from build123d import *

# Parameters (mm, degrees)
SKETCH1_W               = 8
SKETCH1_H               = 8
BOSS_EXTRUDE1_DEPTH     = 3
CUT_EXTRUDE1_DEPTH      = 12.704699911
CUT_EXTRUDE1_DEPTH_BACK = 12.704699911
CUT_EXTRUDE2_DEPTH      = 11
SKETCH4_R               = 1.8
CUT_EXTRUDE3_DEPTH      = 0.8
SKETCH5_W               = 8
SKETCH5_H               = 1
BOSS_EXTRUDE2_DEPTH     = 2
FILLET1_R               = 4
CUT_EXTRUDE4_DEPTH      = 0.4
CUT_EXTRUDE5_DEPTH      = 0.4


with BuildPart() as part:
    # Sketch1 → Boss-Extrude1 (new body)
    with BuildSketch(Plane(origin=(0, 0, 0), x_dir=(1, 0, 0), z_dir=(0, 1, 0))):
        with Locations((4, 4)):
            Rectangle(SKETCH1_W, SKETCH1_H)
    extrude(amount=BOSS_EXTRUDE1_DEPTH)

    # Sketch2 → Cut-Extrude1 (cut, two sides: drawn at the far end of the back side and taken through both)
    with BuildSketch(Plane.XY.offset(-CUT_EXTRUDE1_DEPTH_BACK)):
        Polygon((0, 0), (0.6, 3), (0, 3), align=None)
        Polygon((8, 0), (7.4, 3), (8, 3), align=None)
    extrude(amount=CUT_EXTRUDE1_DEPTH + CUT_EXTRUDE1_DEPTH_BACK, mode=Mode.SUBTRACT)

    # Sketch3 → Cut-Extrude2 (cut)
    with BuildSketch(Plane(origin=(0, 0, 0), x_dir=(0, 0, -1), z_dir=(1, 0, 0))):
        Polygon((0, 0), (0.6, 3), (0, 3), align=None)
        Polygon((8, 3), (7.4, 3), (8, 0), align=None)
    extrude(amount=CUT_EXTRUDE2_DEPTH, mode=Mode.SUBTRACT)

    # Sketch4 → Cut-Extrude3 (cut)
    with BuildSketch(Plane.XZ):
        with Locations(Location((4, -3.75, 0), (0, 0, 270))):
            Circle(SKETCH4_R)
    extrude(amount=-CUT_EXTRUDE3_DEPTH, mode=Mode.SUBTRACT)

    # Sketch5 → Boss-Extrude2 (add)
    with BuildSketch(Plane.XZ):
        with Locations((4, -7.5)):
            Rectangle(SKETCH5_W, SKETCH5_H)
    extrude(amount=BOSS_EXTRUDE2_DEPTH)

    # Fillet1
    # the kernel refuses this fillet: 4 mm, written as the material it takes off along each edge
    with BuildSketch(Plane(origin=(8, -2, -16.660254038), x_dir=(0, 1, 0), z_dir=(0, 0, 1)), Plane(origin=(0, -2, 1.660254038), x_dir=(0, 1, 0), z_dir=(0, 0, -1))) as fillet1_piece_1:
        with BuildLine():
            CenterArc((4, 3.464101615), FILLET1_R, 180, 60)
            Line((0, 3.464101615), (-0.08, 3.464101615))
            Line((-0.08, 3.464101615), (-0.08, 0))
            Line((-0.08, 0), (0, -0.08))
            ThreePointArc((0, -0.08), (1, -0.08), (1.96, -0.069282032))
            Line((1.96, -0.069282032), (2, 0))
        make_face()
    extrude(amount=18.320508076, mode=Mode.SUBTRACT)

    # Sketch6 → Cut-Extrude4 (cut)
    with BuildSketch(Plane(origin=(0, 3, 0), x_dir=(1, 0, 0), z_dir=(0, 1, 0))):
        with BuildLine():
            add(Edge.make_bspline(
                [(5.284087955, 2.773445367), (5.333545491, 2.739545524), (5.432652736, 2.671614118), (5.590291823, 2.583736248), (5.752942084, 2.503846486), (5.865979951, 2.460876102), (5.92270975, 2.439310751)],
                knots=[0, 0, 0, 0, 0.994855506, 1.99357661, 2.993045438, 4, 4, 4, 4], degree=3))
            Line((5.92270975, 2.439310751), (5.628639237, 1.875208187))
            add(Edge.make_bspline(
                [(5.628639237, 1.875208187), (5.568520037, 1.893818156), (5.447325875, 1.93133395), (5.332925255, 1.986187111), (5.275273852, 2.013829982)],
                knots=[0, 0, 0, 0, 0.992113803, 2, 2, 2, 2], degree=3))
            add(Edge.make_bspline(
                [(5.275273852, 2.013829982), (5.26961656, 2.016684314), (5.253233801, 2.024950075), (5.223476786, 2.045298413), (5.178074812, 2.072724498), (5.118973761, 2.11071311), (5.045578888, 2.157800121), (4.95765273, 2.213934729), (4.856407872, 2.280704114), (4.783596416, 2.327731001), (4.744825134, 2.35277229)],
                knots=[0, 0, 0, 0, 0.241377655, 0.698997227, 1.371388316, 2.263975901, 3.376788369, 4.695767198, 6.240533187, 8, 8, 8, 8], degree=3))
            add(Edge.make_bspline(
                [(4.744825134, 2.35277229), (4.712670389, 2.339001865), (4.648050063, 2.311327899), (4.547788838, 2.27725121), (4.444978029, 2.248544986), (4.339982896, 2.224200245), (4.232359046, 2.206111381), (4.122258624, 2.192239309), (4.00937299, 2.18410397), (3.933139287, 2.183304154), (3.894664878, 2.182900495)],
                knots=[0, 0, 0, 0, 0.961025642, 1.931341354, 2.907359807, 3.893838693, 4.891829695, 5.905170566, 6.942759923, 8, 8, 8, 8], degree=3))
            add(Edge.make_bspline(
                [(3.894664878, 2.182900495), (3.821683976, 2.184676763), (3.679027131, 2.188148859), (3.471015208, 2.212756542), (3.275562804, 2.255408477), (3.091812023, 2.313667662), (2.920867424, 2.390147666), (2.761229426, 2.482594503), (2.615108223, 2.593406711), (2.480490537, 2.71918809), (2.361392609, 2.861354588), (2.257130725, 3.017424584), (2.168806746, 3.186880722), (2.097587685, 3.370615377), (2.041301668, 3.567142879), (2.002926315, 3.777850586), (1.978227581, 4.001488849), (1.975427333, 4.155321196), (1.973991801, 4.234182546)],
                knots=[0, 0, 0, 0, 1.098101164, 2.146474535, 3.146072545, 4.104420533, 5.041773038, 5.958565538, 6.874115049, 7.795336865, 8.725215067, 9.658214839, 10.614563411, 11.594512188, 12.618591104, 13.685899083, 14.813688224, 16, 16, 16, 16], degree=3))
            add(Edge.make_bspline(
                [(1.973991801, 4.234182546), (1.97543059, 4.313040679), (1.978227497, 4.466335509), (2.002757559, 4.689542909), (2.042412611, 4.899497801), (2.098124704, 5.096337583), (2.170410456, 5.279545107), (2.259079723, 5.449017762), (2.363505524, 5.605417057), (2.484015277, 5.747270094), (2.617919267, 5.874338646), (2.764464989, 5.984327234), (2.9219486, 6.078236158), (3.090996271, 6.154643933), (3.272074664, 6.212871015), (3.463805003, 6.255387163), (3.667248709, 6.280295733), (3.806454886, 6.283712517), (3.877837955, 6.285464598)],
                knots=[0, 0, 0, 0, 1.193283781, 2.319662245, 3.393996131, 4.424093603, 5.411284417, 6.369670503, 7.313761776, 8.251713527, 9.181123148, 10.102053383, 11.01932051, 11.951118596, 12.903560284, 13.893239571, 14.919681386, 16, 16, 16, 16], degree=3))
            add(Edge.make_bspline(
                [(3.877837955, 6.285464598), (3.948708316, 6.284176334), (4.086935049, 6.281663683), (4.288489067, 6.254790298), (4.478939684, 6.214016744), (4.658513444, 6.155241629), (4.826290277, 6.078911265), (4.983143341, 5.98623667), (5.128157857, 5.876434989), (5.26137487, 5.750578969), (5.380523981, 5.609215368), (5.486073462, 5.454669187), (5.572731816, 5.285035211), (5.645736122, 5.103191508), (5.700157026, 4.90736457), (5.740330715, 4.69867705), (5.764520815, 4.476471411), (5.76739165, 4.323719862), (5.768863596, 4.245400495)],
                knots=[0, 0, 0, 0, 1.078752742, 2.104017338, 3.091035458, 4.041673215, 4.975566109, 5.892967701, 6.810684895, 7.740128604, 8.678185021, 9.621404646, 10.583875016, 11.573429805, 12.6009998, 13.674031063, 14.80742018, 16, 16, 16, 16], degree=3))
            add(Edge.make_bspline(
                [(5.768863596, 4.245400495), (5.767275795, 4.16278925), (5.764189157, 4.002195454), (5.737326284, 3.768977018), (5.693780668, 3.550562854), (5.648918616, 3.41330904), (5.627036673, 3.346362034)],
                knots=[0, 0, 0, 0, 1.083667057, 2.106616435, 3.076482036, 4, 4, 4, 4], degree=3))
            add(Edge.make_bspline(
                [(5.627036673, 3.346362034), (5.607421404, 3.297050064), (5.567517691, 3.196733787), (5.488642668, 3.051933408), (5.394797316, 2.909076479), (5.321514211, 2.819296637), (5.284087955, 2.773445367)],
                knots=[0, 0, 0, 0, 0.948216854, 1.928975575, 2.942311585, 4, 4, 4, 4], degree=3))
        make_face()
        with BuildLine():
            add(Edge.make_bspline(
                [(4.642261032, 3.185304341), (4.671182259, 3.216922768), (4.72909393, 3.280235293), (4.800707281, 3.388678336), (4.863230922, 3.50497094), (4.912388312, 3.632014464), (4.951923574, 3.76787431), (4.97951585, 3.913560578), (4.996652709, 4.068707035), (4.998621406, 4.175375245), (4.999632827, 4.230176136)],
                knots=[0, 0, 0, 0, 0.906820982, 1.815812261, 2.745108282, 3.70056618, 4.696560745, 5.740060838, 6.83895416, 8, 8, 8, 8], degree=3))
            add(Edge.make_bspline(
                [(4.999632827, 4.230176136), (4.998745764, 4.286560817), (4.997027382, 4.395786947), (4.982794262, 4.554398979), (4.957747484, 4.70183414), (4.925058455, 4.838707416), (4.88052022, 4.963910999), (4.826807351, 5.078388614), (4.763835344, 5.182421929), (4.690056733, 5.274294514), (4.608907177, 5.355063587), (4.522159409, 5.426414517), (4.428546166, 5.486139657), (4.328544236, 5.534184829), (4.222990468, 5.571989212), (4.111634776, 5.59943433), (3.994225982, 5.615495039), (3.913944994, 5.6176829), (3.873030263, 5.618797931)],
                knots=[0, 0, 0, 0, 1.335693338, 2.587451293, 3.768164612, 4.876224393, 5.916940853, 6.910477009, 7.867661778, 8.790666633, 9.694493319, 10.576027549, 11.446684429, 12.318352473, 13.199023277, 14.098364444, 15.030842682, 16, 16, 16, 16], degree=3))
            add(Edge.make_bspline(
                [(3.873030263, 5.618797931), (3.831841607, 5.617719084), (3.751279942, 5.615608947), (3.633755604, 5.599158788), (3.522145798, 5.573035665), (3.416723766, 5.534932642), (3.316536446, 5.486796326), (3.222573421, 5.427181815), (3.134847786, 5.356951252), (3.053289548, 5.276692152), (2.980446173, 5.184790487), (2.915694165, 5.082568667), (2.862164439, 4.968850144), (2.819178201, 4.84427298), (2.784825228, 4.709477379), (2.760087026, 4.563739976), (2.745835322, 4.407279692), (2.744110931, 4.299383286), (2.74322257, 4.243797931)],
                knots=[0, 0, 0, 0, 0.980107447, 1.917010591, 2.819119613, 3.703969481, 4.579773866, 5.459928929, 6.346604172, 7.250235365, 8.177620171, 9.131899985, 10.124404622, 11.161948974, 12.264485933, 13.431998172, 14.677033863, 16, 16, 16, 16], degree=3))
            add(Edge.make_bspline(
                [(2.74322257, 4.243797931), (2.744089067, 4.187408458), (2.745771696, 4.077907007), (2.760333697, 3.91913972), (2.783941374, 3.771215716), (2.817547327, 3.634196218), (2.86051391, 3.507924697), (2.913437174, 3.392577112), (2.976036542, 3.288297709), (3.048513511, 3.196032652), (3.128245057, 3.114861766), (3.213441608, 3.04409835), (3.303411645, 2.983479498), (3.39857486, 2.934226809), (3.498956775, 2.896402137), (3.604207339, 2.869103357), (3.714939061, 2.852831885), (3.790443662, 2.850669982), (3.82895975, 2.849567162)],
                knots=[0, 0, 0, 0, 1.356840463, 2.634818045, 3.833173645, 4.958776583, 6.025986406, 7.038359119, 8.007356852, 8.946032033, 9.855123386, 10.740685277, 11.607120956, 12.460971081, 13.313368256, 14.183325659, 15.073285775, 16, 16, 16, 16], degree=3))
            add(Edge.make_bspline(
                [(3.82895975, 2.849567162), (3.857844622, 2.850073951), (3.914741814, 2.851072222), (3.998801079, 2.862293633), (4.080683558, 2.878515583), (4.133570622, 2.895033243), (4.159889237, 2.903253059)],
                knots=[0, 0, 0, 0, 1.028828871, 2.026578908, 3.017950568, 4, 4, 4, 4], degree=3))
            add(Edge.make_bspline(
                [(4.159889237, 2.903253059), (4.119539232, 2.924336443), (4.039635796, 2.966086993), (3.916101198, 3.019284802), (3.792319766, 3.067214804), (3.708133251, 3.09310976), (3.666299493, 3.105977418)],
                knots=[0, 0, 0, 0, 1.021704821, 2.023239566, 3.017713044, 4, 4, 4, 4], degree=3))
            Line((3.666299493, 3.105977418), (3.889857186, 3.56751588))
            add(Edge.make_bspline(
                [(3.889857186, 3.56751588), (3.955233958, 3.544923565), (4.086618506, 3.49952088), (4.276409331, 3.409366748), (4.463555304, 3.306758821), (4.582244486, 3.226093623), (4.642261032, 3.185304341)],
                knots=[0, 0, 0, 0, 0.979271047, 1.967993817, 2.972492781, 4, 4, 4, 4], degree=3))
        make_face(mode=Mode.SUBTRACT)
    extrude(amount=-CUT_EXTRUDE4_DEPTH, mode=Mode.SUBTRACT)

    # Sketch7 → Cut-Extrude5 (cut)
    with BuildSketch(Plane(origin=(0, 3, 0), x_dir=(1, 0, 0), z_dir=(0, 1, 0))):
        with BuildLine():
            Line((6.989609495, 0.992731968), (6.662686419, 0.992731968))
            Line((6.662686419, 0.992731968), (6.662686419, 2.203028442))
            add(Edge.make_bspline(
                [(6.662686419, 2.203028442), (6.647868508, 2.187985499), (6.618433709, 2.158103687), (6.571421698, 2.116422543), (6.522616062, 2.07764809), (6.471533827, 2.042148614), (6.418842766, 2.009418309), (6.364004407, 1.979715431), (6.307416238, 1.952628999), (6.268215163, 1.937491891), (6.248583854, 1.929911455)],
                knots=[0, 0, 0, 0, 1.012567276, 2.011397996, 3.011400399, 4.000747768, 4.993445519, 5.985067596, 6.990952157, 8, 8, 8, 8], degree=3))
            Line((6.248583854, 1.929911455), (6.248583854, 2.256834532))
            add(Edge.make_bspline(
                [(6.248583854, 2.256834532), (6.270355964, 2.264998139), (6.315923296, 2.282083933), (6.383165354, 2.318426283), (6.453350876, 2.363421778), (6.512310721, 2.40755194), (6.559122414, 2.44678718), (6.591840229, 2.478326157), (6.622155165, 2.510623705), (6.648927745, 2.544722271), (6.672860762, 2.579932457), (6.694066458, 2.616196741), (6.712732345, 2.65362968), (6.722503807, 2.679697149), (6.727389944, 2.692731968)],
                knots=[0, 0, 0, 0, 1.253673617, 2.623841347, 4.114270668, 5.751233548, 6.594491912, 7.409089316, 8.202422231, 8.983165545, 9.746111525, 10.498431446, 11.249153235, 12, 12, 12, 12], degree=3))
            Line((6.727389944, 2.692731968), (6.989609495, 2.692731968))
            Line((6.989609495, 2.692731968), (6.989609495, 0.992731968))
        make_face()
    extrude(amount=-CUT_EXTRUDE5_DEPTH, mode=Mode.SUBTRACT)


solid = part.part
Design review of the part built by this model. Coordinates are the model's own, in mm. A direction names the side the tool comes from. Round coordinates to 2 decimals unless told otherwise and drop trailing zeros. Order: outer loops, then holes, each group sorted by start corner. A loop starts at its lowest first (then second) coordinate and runs counter-clockwise, first axis right, second up. Notation, with made-up numbers: M -33.75,80 L 8.25,80 A24 cw 8.25,91 Z; hole C -17.5,78 d1. An arc over 180 degrees is marked long. Answer as CSV lines item,"result". Start each with the question number.
1) Wall thickness on line 1 along Y through (x, z) = (5.5, -0.75); line 2 along X through (y, z) = (0.55, -3.75); line 3 along Y through (x, z) = (5, -5.75): over which ranges is each line inside the solid? List them lowest first. Write a range as [from, to].
2) Add section A-A (y = 0.2). Give the boundary of the cut face in (x, z).
3) The part is to be moulded in two halves that separate along Z. For faces 6 (the face through (6.51, -1.48, -7.51)), 7 (the face through (4, -1, -8)), 8 (the face through (4, 0.8, -4)), say which applies: +Z half, -Z half, draft (parallel to the pull), parting line (faces both ways), or undercut.
4) Add section D-D (y = 2.3). Give the boundary of the cut face in (x, z), then the cut area to 3 significant figures.
5) Add section C-C (x = 7.5). Give the boundary of the cut face in (y, z), then the cut area to 3 significant figures.
6) Add section B-B (z = -7.25). Give the boundary of the cut face in (x, y).
7) For pin 1 Ø2 at (x, z) = (6.5, -3.5) entering from -Y; pin 2 Ø1.8 at (x, z) = (4, -4.5) entering from -Y; pin 3 Ø2 at (y, z) = (1.5, -5.5) entering from -X, all flat-tipped, find the tip position at first contact; note any pin that passes through.
8) Tool access review of faces 1 (the face through (4.541, 0.394, -5.467)), 2 (the face through (4, 3, -4)), 3 (the face through (3.9, 1.5, -7.7)), 4 (the face through (4, -1, -7)), 5 (the face through (4.4, 2.6, -3.1)): name each direction out of +Z, -Z, +X, -X, +Y, -Y from which nothing blocks a thin tool from reaching the whole face with its end or side.
Resolved:
1,line 1,"[0, 3]"
1,line 2,"[0.11, 2.2], [5.8, 7.89]"
1,line 3,"[0, 2.6]"
2,outline,"M 0.04,-7.96 L 7.96,-7.96 L 7.96,-0.04 L 0.04,-0.04 Z; hole C 4,-3.75 d3.6"
3,face 6,"draft"
3,face 7,"-Z half"
3,face 8,"undercut"
4,outline,"M 0.46,-7.54 L 7.54,-7.54 L 7.54,-0.46 L 0.46,-0.46 Z"
4,area,"50.1 mm^2"
5,outline,"M -0.69,-8 L 0,-8 L 2.5,-7.5 L 2.5,-0.5 L 0,0 L 0,-7 L -0.69,-7 Z"
5,area,"19.4 mm^2"
6,outline,"M 0,0 A4 ccw 3.46,-2 L 4.54,-2 A4 ccw 8,0 L 7.4,3 L 0.6,3 Z"
7,pin 1,"y = 0"
7,pin 2,"y = 0.8"
7,pin 3,"x = 0.1"
8,face 1,"-Y"
8,face 2,"+Z, -Z, +X, -X, +Y"
8,face 3,"-Z, +X, -X, +Y"
8,face 4,"+Z, +X, -X, -Y"
8,face 5,"+Y"
